```python
from build123d import *

# Parameters (mm, degrees)
SKETCH_4_W = 0.4
SKETCH_4_H = 0.4


with BuildPart() as part:
    # По траектории1: sweep along a curve in space
    with BuildLine() as sweep_1_path:
        Line((0, 0, 0), (0, 0, -13.1))
        Line((0, 0, -13.1), (0, 5, -13.1))
    # Эскиз4 → По траектории1 (sweep)
    with BuildSketch(Plane.XY):
        Rectangle(SKETCH_4_W, SKETCH_4_H)
    sweep(path=sweep_1_path.line, transition=Transition.RIGHT)


solid = part.part
```
Design review of the part built by this model. Coordinates are the model's own, in mm. Coordinates: 2 decimals unless noted, no trailing zeros. Write each loop counter-clockwise with the first axis right and the second up, starting at its lowest first coordinate (ties: lowest second). Pieces come first, ordered by that corner, then holes.
1) Add section C-C (y = 2.3). Write out the cut boundary in (x, z).
2) To check wall thickness, follow L1, parallel to Z at x = 0.05, y = 2.65; L2, parallel to Y at x = 0.15, z = -1. State the ranges of each line that lie inside material, in increasing order.
3) Add section A-A (x = -0.1). Write out the cut boundary in (y, z), plus the area to 3 significant figures.
4) Add section B-B (z = -8.75). Write out the cut boundary in (x, y), plus the area to 3 significant figures.
Check result:
1. outline: (-0.2, -13.3) - (0.2, -13.3) - (0.2, -12.9) - (-0.2, -12.9) - close
2. L1: z = -13.3 to -12.9
2. L2: y = -0.2 to 0.2
3. outline: (-0.2, -13.3) - (5, -13.3) - (5, -12.9) - (0.2, -12.9) - (0.2, 0) - (-0.2, 0) - close
3. area: 7.24 mm2
4. outline: (-0.2, -0.2) - (0.2, -0.2) - (0.2, 0.2) - (-0.2, 0.2) - close
4. area: 0.160 mm2
